from build123d import *

# Parameters (mm, degrees)
SKETCH1_R                  = 67.5
BOSS_EXTRUDE1_DEPTH        = 10
CUT_EXTRUDE1_DEPTH         = 96.981769102
CUT_EXTRUDE1_DEPTH_BACK    = 96.981769102
SKETCH4_R                  = 4
CUT_EXTRUDE_THIN1_DEPTH    = 96.981769102
F_5_0MM_DOWEL_HOLE1_REACH  = 162.34
F_5_0MM_DOWEL_HOLE1_BORE_R = 2.5
CIRPATTERN1_COUNT          = 4
F_3_0MM_DOWEL_HOLE1_D      = 3
CUT_EXTRUDE2_DEPTH         = 96.981769113
CUT_EXTRUDE2_DEPTH_BACK    = 96.981769113
SKETCH13_R                 = 11.25


with BuildPart() as part:
    # Sketch1 → Boss-Extrude1 (new body)
    with BuildSketch(Plane(origin=(0, 0, 0), x_dir=(1, 0, 0), z_dir=(0, 1, 0))):
        with Locations(Location((0, 0, 0), (0, 0, 270))):
            Circle(SKETCH1_R)
    extrude(amount=BOSS_EXTRUDE1_DEPTH)

    # Sketch4 → Cut-Extrude1 (cut, two sides: drawn at the far end of the back side and taken through both)
    with BuildSketch(Plane(origin=(0, 10, 0), x_dir=(1, 0, 0), z_dir=(0, 1, 0)).offset(-CUT_EXTRUDE1_DEPTH_BACK)):
        with Locations(Location((-40, 40, 0), (0, 0, 270))):
            Circle(SKETCH4_R)
        with Locations(Location((40, 40, 0), (0, 0, 270))):
            Circle(SKETCH4_R)
        with Locations(Location((40, -40, 0), (0, 0, 270))):
            Circle(SKETCH4_R)
        with Locations(Location((-40, -40, 0), (0, 0, 270))):
            Circle(SKETCH4_R)
    extrude(amount=CUT_EXTRUDE1_DEPTH + CUT_EXTRUDE1_DEPTH_BACK, mode=Mode.SUBTRACT)

    # Sketch5 → Cut-Extrude-Thin1 (cut, through all)
    with BuildSketch(Plane(origin=(0, 10, 0), x_dir=(1, 0, 0), z_dir=(0, 1, 0))):
        Polygon((-31.743671291, 59.570037208), (-59.570037208, 31.743671291), (-66.64110502, 38.814739103), (-38.814739103, 66.64110502), align=None)
        Polygon((59.570037208, 31.743671291), (31.743671291, 59.570037208), (38.814739103, 66.64110502), (66.64110502, 38.814739103), align=None)
        Polygon((31.743671291, -59.570037208), (59.570037208, -31.743671291), (66.64110502, -38.814739103), (38.814739103, -66.64110502), align=None)
        Polygon((-59.570037208, -31.743671291), (-31.743671291, -59.570037208), (-38.814739103, -66.64110502), (-66.64110502, -38.814739103), align=None)
    extrude(amount=-CUT_EXTRUDE_THIN1_DEPTH, mode=Mode.SUBTRACT)

    # Ø5.0mm Dowel Hole1 bore → Ø5.0mm Dowel Hole1 (cut, up to next)
    with BuildSketch(Plane(origin=(45.656854249, 0, 45.656854249), x_dir=(0.7071067811865479, 0, -0.7071067811865471), z_dir=(0.7071067811865471, 0, 0.7071067811865479)), mode=Mode.PRIVATE) as f_5_0mm_dowel_hole1_sk1:
        with Locations((0, 5)):
            Circle(F_5_0MM_DOWEL_HOLE1_BORE_R)
    f_5_0mm_dowel_hole1_tool1 = extrude(f_5_0mm_dowel_hole1_sk1.sketch, amount=-F_5_0MM_DOWEL_HOLE1_REACH, mode=Mode.PRIVATE) & part.part
    f_5_0mm_dowel_hole1 = f_5_0mm_dowel_hole1_tool1.solids().sort_by_distance((45.656854, 5, 45.656854))[0]
    add(f_5_0mm_dowel_hole1, mode=Mode.SUBTRACT)

    # CirPattern1: Ø5.0mm Dowel Hole1 ×4 about axis
    cirpattern1_axis = Axis((0, 10, 0), (0, -1, 0))
    for i in range(1, CIRPATTERN1_COUNT):
        add(f_5_0mm_dowel_hole1.rotate(cirpattern1_axis, i * 360 / CIRPATTERN1_COUNT), mode=Mode.SUBTRACT)

    # Ø3.0mm Dowel Hole1 (through all)
    with Locations(Plane(origin=(0, 0, 0), x_dir=(-1, 0, 0), z_dir=(0, -1, 0))):
        with Locations((0, 21.920310217), (21.920310217, 0), (-21.920310217, 0), (0, -21.920310217)):
            Hole(F_3_0MM_DOWEL_HOLE1_D / 2)

    # Sketch13 → Cut-Extrude2 (cut, two sides: drawn at the far end of the back side and taken through both)
    with BuildSketch(Plane(origin=(0, 10, 0), x_dir=(1, 0, 0), z_dir=(0, 1, 0)).offset(-CUT_EXTRUDE2_DEPTH_BACK)):
        with Locations(Location((0, 0, 0), (0, 0, 270))):
            Circle(SKETCH13_R)
    extrude(amount=CUT_EXTRUDE2_DEPTH + CUT_EXTRUDE2_DEPTH_BACK, mode=Mode.SUBTRACT)


solid = part.part
Design review of the part built by this model. Coordinates are the model's own, in mm. Coordinates: 2 decimals unless noted, no trailing zeros. Order: outer loops, then holes, each group sorted by start corner. A loop starts at its lowest first (then second) coordinate and runs counter-clockwise, first axis right, second up. Notation, with made-up numbers: (53, 41) -> (101, 41) arc R33 cw to (101, 77) -> close; hole circle Ø7 at (-5, 13). An arc over 180 degrees is marked (long way). Use one line per item in the form item = value. Start each with the question number.
(1) Add section B-B on z = -6. State the section outline as (x, y) points, plus the area to 3 significant figures.
(2) The part is to be moulded in two halves that separate along Y. For faces 1 (the flat face through (45.852, 8.403, -45.462)), 2 (the flat face through (-14, 0, -1)), 3 (the cylindrical face through (43.14, 2.78, -44.77)), say which applies: +Y half, -Y half, draft (parallel to the pull), parting line (faces both ways), or undercut.
(3) Add section C-C on x = -54.5. State the section outline as (y, z) points.
(4) Insertion check: pin 1 (6.5 mm diameter, centred on x = -40, z = -40, fed in from -Y); pin 2 (1.5 mm diameter, centred on y = 3, z = -37, fed in from +X); pin 3 (6 mm diameter, centred on x = -1, y = 7.5, fed in from -Z); pin 4 (1.5 mm diameter, centred on y = 1.5, z = 1, fed in from -X). Each pin has a flat end and moves straight along its axis. Give the tip position at first contact, or say it passes through.
(5) Add section D-D on z = 57. State the section outline as (x, y) points.
(6) Add section A-A on x = 9. State the section outline as (y, z) points, plus the area to 3 significant figures.
(7) For probe 1 along Z at (x, y) = (0, 6.5); probe 2 along X at (y, z) = (8, 40); probe 3 along Z at (x, y) = (43, 4.75), list the stretches that pass through material, from the lowest coordinate up.
Answer block:
q1.outline = (-67.23, 0) -> (-9.52, 0) -> (-9.52, 10) -> (-67.23, 10) -> close; (9.52, 0) -> (67.23, 0) -> (67.23, 10) -> (9.52, 10) -> close
q1.area = 1,150 mm²
q2.face_1 = draft
q2.face_2 = -Y half
q2.face_3 = undercut
q3.outline = (0, -36.81) -> (10, -36.81) -> (10, 36.81) -> (0, 36.81) -> close
q4.pin_1 = through
q4.pin_2 = 55.06
q4.pin_3 = -67.5
q4.pin_4 = -67.5
q5.outline = (-34.31, 0) -> (34.31, 0) -> (34.31, 10) -> (-34.31, 10) -> close
q6.outline = (0, -66.9) -> (10, -66.9) -> (10, -6.75) -> (0, -6.75) -> close; (0, 6.75) -> (10, 6.75) -> (10, 66.9) -> (0, 66.9) -> close
q6.area = 1,200 mm²
q7.probe_1 = -67.5 to -23.42, -20.42 to -11.25, 11.25 to 20.42, 23.42 to 67.5
q7.probe_2 = -51.31 to -44, -36 to 36, 44 to 51.31
q7.probe_3 = -48.31 to -46.52, -37.35 to 37.35, 46.52 to 48.31
